from build123d import *

# Parameters (mm, degrees)
SKETCH1_R            = 19.8
GEARBOX_DEPTH        = 24.25
SKETCH2_R            = 16.75
MOTOR_DEPTH          = 40
SKETCH3_R            = 18.3
GEARBOX_LIP_DEPTH    = 2.5
SKETCH4_R            = 6
SHAFT_HUB_DEPTH      = 5.6
SHAFT_DEPTH          = 15
SKETCH6_R            = 1.5
MNT_SCREW_HOLE_DEPTH = 4
CIRPATTERN1_COUNT    = 6
SKETCH7_R            = 1
SENSORSHAFT_DEPTH    = 7


with BuildPart() as part:
    # Sketch1 → gearbox (new body)
    with BuildSketch(Plane.XY):
        with Locations(Location((0, 0, 0), (0, 0, 180))):
            Circle(SKETCH1_R)
    extrude(amount=GEARBOX_DEPTH)

    # Sketch2 → motor (add)
    with BuildSketch(Plane.XY.offset(24.25)):
        Circle(SKETCH2_R)
    extrude(amount=MOTOR_DEPTH)

    # Sketch3 → gearbox lip (add)
    with BuildSketch(Plane(origin=(0, 0, 0), x_dir=(-1, 0, 0), z_dir=(0, 0, -1))):
        Circle(SKETCH3_R)
    extrude(amount=GEARBOX_LIP_DEPTH)

    # Sketch4 → shaft hub (add)
    with BuildSketch(Plane(origin=(0, 0, -2.5), x_dir=(-1, 0, 0), z_dir=(0, 0, -1))):
        with Locations((0, 7)):
            Circle(SKETCH4_R)
    extrude(amount=SHAFT_HUB_DEPTH)

    # Sketch5 → shaft (add)
    with BuildSketch(Plane(origin=(0, 0, -8.1), x_dir=(-1, 0, 0), z_dir=(0, 0, -1))):
        with BuildLine():
            Line((-1.71537168, 4.6), (1.71537168, 4.6))
            ThreePointArc((1.71537168, 4.6), (0, 9.95), (-1.71537168, 4.6))
        make_face()
    extrude(amount=SHAFT_DEPTH)

    # Sketch6 → mnt screw hole (cut)
    with BuildSketch(Plane(origin=(0, 0, -2.5), x_dir=(-1, 0, 0), z_dir=(0, 0, -1))):
        with Locations((-15.5, 0)):
            Circle(SKETCH6_R)
    mnt_screw_hole = extrude(amount=-MNT_SCREW_HOLE_DEPTH, mode=Mode.SUBTRACT)

    # CirPattern1: mnt screw hole ×6 about axis
    cirpattern1_axis = Axis((0, 0, 0), (0, 0, 1))
    for i in range(1, CIRPATTERN1_COUNT):
        add(mnt_screw_hole.rotate(cirpattern1_axis, i * 360 / CIRPATTERN1_COUNT), mode=Mode.SUBTRACT)

    # Sketch7 → sensorshaft (add)
    with BuildSketch(Plane.XY.offset(64.25)):
        Circle(SKETCH7_R)
    extrude(amount=SENSORSHAFT_DEPTH)


solid = part.part
Verification items for the finished model (mm, model axes). A direction names the side the tool comes from. Give positions to 0.01 mm unless a question says otherwise; leave off trailing zeros. Loops run counter-clockwise (first coordinate to the right, second up) from the corner with the lowest first, then second, coordinate; pieces in that order, holes last. Notation, with made-up numbers: (38, 29) - (68, 29) arc R33 ccw to (68, 66) - close; hole circle Ø8 at (-15.75, 33.25). An arc over 180 degrees is marked (long way). Write each question's results on one line, items separated by ' | '.
1) Material ranges on L1, parallel to Y at x = -7.75, z = 0.45; L2, parallel to Z at x = 11, y = -11; L3, parallel to Z at x = 8, y = -13.5, recorded low to high. Write a range as from..to.
Solution:
L1: -18.22..-14.92, -11.92..11.92, 14.92..18.22 | L2: -2.5..64.25 | L3: 1.5..64.25
2) Depth check by flat-ended pin: P1, Ø4, axis at y = 3, z = 7.5, coming from the -X side; P2, Ø4, axis at x = 7.75, y = -13.42, coming from the +Z side; P3, Ø3.5, axis at x = 7.5, y = 13.5, coming from the -Z side. Enter the tip coordinate at first touch or a pass-through.
Solution:
P1: x = -19.77 | P2: z = 64.25 | P3: z = -2.5
3) Sectioned sample at B-B on y = 0. Record the boundary of the cut face in (x, z).
Solution:
outline: (-19.8, 0) - (-18.3, 0) - (-18.3, -2.5) - (-17, -2.5) - (-17, 1.5) - (-14, 1.5) - (-14, -2.5) - (14, -2.5) - (14, 1.5) - (17, 1.5) - (17, -2.5) - (18.3, -2.5) - (18.3, 0) - (19.8, 0) - (19.8, 24.25) - (16.75, 24.25) - (16.75, 64.25) - (1, 64.25) - (1, 71.25) - (-1, 71.25) - (-1, 64.25) - (-16.75, 64.25) - (-16.75, 24.25) - (-19.8, 24.25) - close
4) Tool access check on faces 1 (the flat face through (0, 4.6, -15)), 2 (the flat face through (15, -9, 24.25)), 3 (the flat face through (-8, -13, 1.5)). Record the directions out of +Z, -Z, +X, -X, +Y, -Y that give a thin tool (end or side, any length) a straight path to the whole face; none if there is none.
Solution:
face 1: -Z, +X, -X, -Y | face 2: +Z | face 3: -Z
5) Sectioned sample at A-A on x = 0. Record the boundary of the cut face in (y, z), plus the area to 3 significant figures.
Solution:
outline: (-19.8, 0) - (-18.3, 0) - (-18.3, -2.5) - (1, -2.5) - (1, -8.1) - (4.6, -8.1) - (4.6, -23.1) - (9.95, -23.1) - (9.95, -8.1) - (13, -8.1) - (13, -2.5) - (18.3, -2.5) - (18.3, 0) - (19.8, 0) - (19.8, 24.25) - (16.75, 24.25) - (16.75, 64.25) - (1, 64.25) - (1, 71.25) - (-1, 71.25) - (-1, 64.25) - (-16.75, 64.25) - (-16.75, 24.25) - (-19.8, 24.25) - close | area: 2,550 mm2
6) Sectioned sample at D-D on z = -15.5. Record the boundary of the cut face in (x, y), plus the area to 3 significant figures.
Solution:
outline: (-1.72, 4.6) - (1.72, 4.6) arc R2.95 ccw (long way) to start | area: 26.1 mm2
7) Sectioned sample at C-C on z = -1. Record the boundary of the cut face in (x, y).
Solution:
outline: circle Ø36.6 at (0, 0); hole circle Ø3 at (-15.5, 0); hole circle Ø3 at (-7.75, -13.42); hole circle Ø3 at (-7.75, 13.42); hole circle Ø3 at (7.75, -13.42); hole circle Ø3 at (7.75, 13.42); hole circle Ø3 at (15.5, 0)
8) Mould release check, pull along X, two halves, no side actions. Record for faces 4 (the flat face through (0, -3, 64.25)), 5 (the cylindrical face through (-8.44, 12.09, -0.53)), 6 (the cylindrical face through (0, -1, 68)): pulls with the +X half, pulls with the -X half, needs draft (parallel to the pull), parting line crosses it, or undercut.
Solution:
face 4: needs draft | face 5: undercut | face 6: parting line crosses it
